```python
from build123d import *

# Parameters (mm, degrees)
F1_DEPTH = 20
F3_DEPTH = 20
F4_W     = 157
F4_H     = 4
F5_DEPTH = 3


with BuildPart() as f1:
    # F0 (on Top) → F1 (new body)
    with BuildSketch(Plane.XY):
        Polygon((0, 187.499995), (-180, 187.499995), (-180, 149.999995), (-160, 149.999995), (-160, 112.499995), (-180, 112.499995), (-180, 74.999995), (-160, 74.999995), (-160, 37.499995), (0, 37.499995), align=None)
    extrude(amount=F1_DEPTH)

    # F2 (on face) → F3 (cut)
    with BuildSketch(Plane.XY.offset(20)):
        Polygon((0, 171.999995), (-20, 176.499995), (-20, 150.499995), (0, 156.999995), align=None)
        Polygon((0, 119.999995), (-20, 125.499995), (-20, 99.499995), (0, 104.999995), align=None)
        Polygon((0, 67.999995), (-20, 74.499995), (-20, 48.499995), (0, 52.999995), align=None)
    extrude(amount=-F3_DEPTH, mode=Mode.SUBTRACT)

    # F4 (on face) → F5 (cut)
    with BuildSketch(Plane(origin=(0, 0, 0), x_dir=(1, 0, 0), z_dir=(0, 0, -1))):
        with Locations((-81.5, -45.499995)):
            Rectangle(F4_W, F4_H)
    extrude(amount=-F5_DEPTH, mode=Mode.SUBTRACT)


solid = f1.part
```
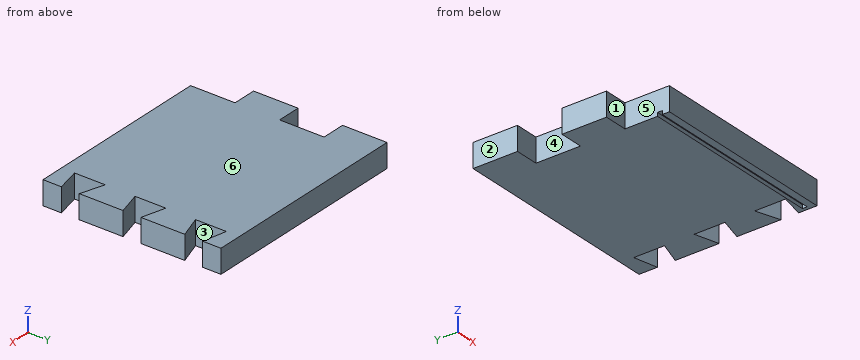
The listing builds one solid part. Answer for the finished solid, in the listing's coordinates (mm). Face numbers are marked on the shaded views. A direction names the side the tool comes from. Coordinates: 2 decimals unless noted, no trailing zeros. Loops run counter-clockwise (first coordinate to the right, second up) from the corner with the lowest first, then second, coordinate; pieces in that order, holes last. Notation, with made-up numbers: (-26.5, -16.5) - (8.5, -16.5) arc R24 ccw to (8.5, -3.5) - close; hole circle Ø5 at (33.5, 61). An arc over 180 degrees is marked (long way). Use a Markdown table: item, result. Add a question column.
1) Find the intervals of material crossed by line 1 (Y direction, x = -26, z = 1); line 2 (X direction, y = 166, z = 5.75); line 3 (X direction, y = 65.5, z = 17.75), in increasing order.
2) The mould has two halves that part along X. Classify the marked faces 1, 2 and 3: released by +X, released by -X, zero draft, split by the parting line, or undercut.
3) For the marked faces 4, 5 and 6, determine the directions among +Z, -Z, +X, -X, +Y, -Y from which every point of the face is accessible in a straight line to the end or side of a thin tool.
4) The part is cut by section D-D, the plane y = 102.5. Give the vertices of the cut face in (x, z), and give its area (3 significant figures).
5) The part is cut by section C-C, the plane y = 63. Give the vertices of the cut face in (x, z).
6) The part is cut by section A-A, the plane z = 12.25. Give the vertices of the cut face in (x, y), and give its area (3 significant figures).
7) The part is cut by section B-B, the plane y = 122.5. Give the vertices of the cut face in (x, z), and give its area (3 significant figures).
8) Given pin 1 (10 mm diameter, centred on y = 62.5, z = 5.5, fed in from -X); pin 2 (10 mm diameter, centred on y = 165.5, z = 13.5, fed in from +X); pin 3 (10 mm diameter, centred on x = -168, z = 11.5, fed in from -Y), each flat-ended and moving along its own axis, determine where each tip first touches the part or whether it passes through.
Here are the results:
| question | item | result |
|---|---|---|
| 1 | line 1 | y = 37.5 to 43.5, 47.5 to 187.5 |
| 1 | line 2 | x = -180 to -20 |
| 1 | line 3 | x = -160 to -20 |
| 2 | face 1 | zero draft |
| 2 | face 2 | released by -X |
| 2 | face 3 | undercut |
| 3 | face 4 | +Z, -Z, -X |
| 3 | face 5 | +Z, -Z, -X, -Y |
| 3 | face 6 | +Z, +X, -X, +Y, -Y |
| 4 | outline | (-180, 0) - (-20, 0) - (-20, 20) - (-180, 20) - close; (-9.09, 0) - (0, 0) - (0, 20) - (-9.09, 20) - close |
| 4 | area | 3,380 mm^2 |
| 5 | outline | (-160, 0) - (-20, 0) - (-20, 20) - (-160, 20) - close |
| 6 | outline | (-180, 75) - (-160, 75) - (-160, 37.5) - (0, 37.5) - (0, 53) - (-20, 48.5) - (-20, 74.5) - (0, 68) - (0, 105) - (-20, 99.5) - (-20, 125.5) - (0, 120) - (0, 157) - (-20, 150.5) - (-20, 176.5) - (0, 172) - (0, 187.5) - (-180, 187.5) - (-180, 150) - (-160, 150) - (-160, 112.5) - (-180, 112.5) - close |
| 6 | area | 24,300 mm^2 |
| 7 | outline | (-160, 0) - (-20, 0) - (-20, 20) - (-160, 20) - close; (-9.09, 0) - (0, 0) - (0, 20) - (-9.09, 20) - close |
| 7 | area | 2,980 mm^2 |
| 8 | pin 1 | stops at x = -160 |
| 8 | pin 2 | stops at x = -20 |
| 8 | pin 3 | stops at y = 75 |
